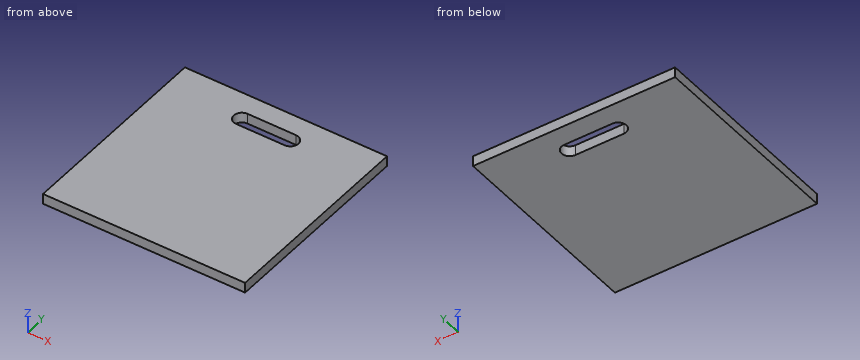
Autodesk Inventor part; units mm, degrees
ref_plane "YZ Plane" through (0, 0, 0) normal (1, 0, 0) x (0, 1, 0)
ref_plane "XZ Plane" through (0, 0, 0) normal (0, 1, 0) x (-1, 0, 0)
ref_plane "XY Plane" through (0, 0, 0) normal (0, 0, 1) x (1, 0, 0)
sketch "Sketch1" plane through (0, 0, 0) normal (0, 0, 1) x (1, 0, 0)
  line L0 (-125, -125) -> (125, -125)
  line L1 (125, -125) -> (125, 125)
  line L2 (125, 125) -> (-125, 125)
  line L3 (-125, 125) -> (-125, -125)
  line L4 (-125, -125) -> (125, 125) construction
  line L5 (125, -125) -> (-125, 125) construction
  point P0 (0, 0)
  dimension "Height" = 250
  dimension "Width" = 250
extrude "Extrusion1" add sketch "Sketch1" along normal blind 12.7
sketch "Sketch2" plane through (0, 0, 12.7) normal (0, 0, 1) x (1, 0, 0)
  line L0 (-30, 90) -> (30, 90) construction
  line L1 (-30, 80) -> (30, 80)
  line L2 (30, 100) -> (-30, 100)
  arc A0 (-30, 100) -> (-30, 80) centre (-30, 90) ccw
  arc A1 (30, 80) -> (30, 100) centre (30, 90) ccw
  line L3 (125, 125) -> (-125, 125)
  point P0 (0, 0)
  point P1 (0, 90)
  dimension "d4" = 30
  dimension "d5" = 20
  dimension "d6" = 25
extrude "Extrusion2" cut sketch "Sketch2" against normal up to surface (12.7 mm away)
equation "\"d7\" = thickness"
properties part number "Creat Front-02" material "Wood (Maple)"
Geometry check sheet. Reference: the model listing, model coordinates, mm. Round coordinates to 2 decimals unless told otherwise and drop trailing zeros. Loops run counter-clockwise (first coordinate to the right, second up) from the corner with the lowest first, then second, coordinate; pieces in that order, holes last. Notation, with made-up numbers: (78.5, -19.5) - (89.5, -19.5) arc R19 cw to (89.5, 13.5) - close; hole circle Ø4 at (29.5, -24.75). An arc over 180 degrees is marked (long way). One line per question, with ' | ' between items. Start each with the question number.
1. Cross-section at B-B on x = 21.5. Record the cut outline in (y, z).
2. Cross-section at A-A on y = 90. Record the cut outline in (x, z), then the cut area to 3 significant figures.
3. Scan lines: line 1 (Y direction, x = -17.5, z = 9.75); line 2 (Y direction, x = 39, z = 1). Record each from-to range of solid material in increasing order. Write a range as [from, to].
4. Depth check by flat-ended pin: pin 1 (12 mm diameter, centred on x = 28, y = 2, fed in from -Z). Enter the tip coordinate at first touch or a pass-through.
5. Cross-section at C-C on z = 6. Record the cut outline in (x, y).
Taken from the geometry:
1) outline: (-125, 0) - (80, 0) - (80, 12.7) - (-125, 12.7) - close; (100, 0) - (125, 0) - (125, 12.7) - (100, 12.7) - close
2) outline: (-125, 0) - (-40, 0) - (-40, 12.7) - (-125, 12.7) - close; (40, 0) - (125, 0) - (125, 12.7) - (40, 12.7) - close | area: 2,160 mm²
3) line 1: [-125, 80], [100, 125] | line 2: [-125, 85.64], [94.36, 125]
4) pin 1: z = 0
5) outline: (-125, -125) - (125, -125) - (125, 125) - (-125, 125) - close; hole (-30, 80) - (30, 80) arc R10 ccw to (30, 100) - (-30, 100) arc R10 ccw to start
